Input: part model. Units: mm. Frame: model coordinates. Face numbers are marked on the shaded views. A direction names the side the tool comes from. Coordinates: 2 decimals unless noted, no trailing zeros. Loops run counter-clockwise (first coordinate to the right, second up) from the corner with the lowest first, then second, coordinate; pieces in that order, holes last. Notation, with made-up numbers: (-27.75, 1) -> (-19.75, 1) arc R33 ccw to (-19.75, 32) -> close; hole circle Ø8 at (6.25, -22). An arc over 180 degrees is marked (long way). Put each result on its own line as item: value. Start each with the question number.
1) Contact query for flat-ended pins moving along their axis: P1, Ø1.5, axis at x = -1, z = 9, coming from the +Y side; P2, Ø2, axis at x = -4.5, z = 47.5, coming from the +Y side; P3, Ø2, axis at y = -81, z = 3.5, coming from the -X side; P4, Ø5, axis at x = -35.5, y = -44, coming from the +Z side. Output: stop coordinate, or through.
2) Cut plane B-B (x = 37.5). Return the cut outline in (y, z), plus the area to 3 significant figures.
3) Cut plane A-A (y = -36.5). Return the cut outline in (x, z), plus the area to 3 significant figures.
4) Material intervals for L1, parallel to X at y = -19, z = 28; L2, parallel to Z at x = -13, y = -70.5, sorted ascending.
5) Cut plane C-C (z = 6). Return the cut outline in (x, y).
6) Cut plane D-D (y = -55.5). Return the cut outline in (x, z).
7) Set-up query: the marked faces 1, 2 and 3. Return all of +Z, -Z, +X, -X, +Y, -Y with unobstructed straight access to the full face (end or side cutting, diameter ignored); none if empty.
from build123d import *

# Parameters (mm, degrees)
F0_W      = 100
F0_H      = 100
F1_DEPTH  = 100
F2_R      = 35
F3_DEPTH  = 70
F4_R      = 35
F5_DEPTH  = 70
F6_R      = 35
F7_DEPTH  = 70
F8_R      = 35
F9_DEPTH  = 70
F11_R     = 35
F12_DEPTH = 70
F13_R     = 35
F14_DEPTH = 25
F10_R     = 35
F15_DEPTH = 70
F17_D     = 5


with BuildPart() as f1:
    # F0 (on Front) → F1 (new body)
    with BuildSketch(Plane.XZ):
        with Locations((50, 50)):
            Rectangle(F0_W, F0_H)
    extrude(amount=F1_DEPTH)

    # F2 (on Top) → F3 (join)
    with BuildSketch(Plane.XY):
        with Locations((48.346177, -50.003812)):
            Circle(F2_R)
    extrude(amount=-F3_DEPTH)

    # F4 (on Top) → F5 (join)
    with BuildSketch(Plane.XY):
        with Locations((49.174994, -45.859754)):
            Circle(F4_R)
    extrude(amount=-F5_DEPTH)

    # F6 (on Top) → F7 (join)
    with BuildSketch(Plane.XY):
        with Locations((48.553377, -49.589396)):
            Circle(F6_R)
    extrude(amount=-F7_DEPTH)

    # F8 (on Top) → F9 (join)
    with BuildSketch(Plane.XY):
        with Locations((50.625414, -48.760593)):
            Circle(F8_R)
    extrude(amount=-F9_DEPTH)

    # F11 (on Top) → F12 (join)
    with BuildSketch(Plane.XY):
        with Locations((50.038069, -49.650535)):
            Circle(F11_R)
    extrude(amount=-F12_DEPTH)

    # F13 (on face) → F14 (join)
    with BuildSketch(Plane.XY.offset(100)):
        with Locations((49.716454, -51.418651)):
            Circle(F13_R)
    extrude(amount=-F14_DEPTH)

    # F10 (on Right) → F15 (join)
    with BuildSketch(Plane.YZ):
        with Locations((-52.281633, 49.393684)):
            Circle(F10_R)
    extrude(amount=-F15_DEPTH)

    # F17 (through all)
    with Locations(Plane.XZ.offset(100)):
        with Locations((50.875958, 50.418209)):
            Hole(F17_D / 2)


solid = f1.part
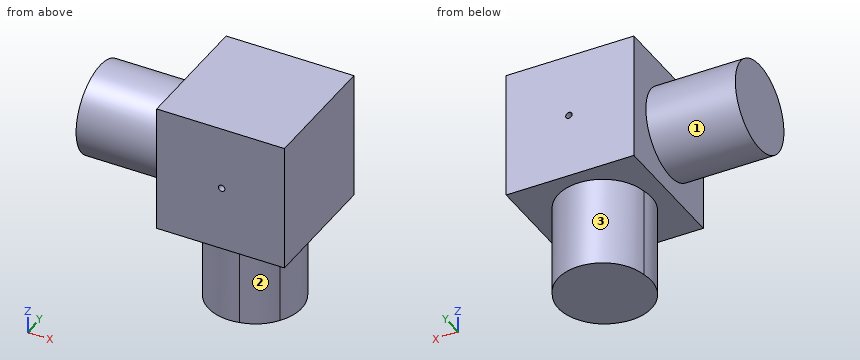
Results found:
1. P1: passes through
1. P2: stops at y = -17.29
1. P3: stops at x = 0
1. P4: stops at z = 83.91
2. outline: (-100, 0) -> (-83.28, 0) -> (-83.28, -70) -> (-12.86, -70) -> (-12.86, 0) -> (0, 0) -> (0, 100) -> (-100, 100) -> close
2. area: 14,900 mm2
3. outline: (-70, 18.15) -> (0, 18.15) -> (0, 0) -> (15.45, 0) -> (15.45, -70) -> (83.41, -70) -> (83.41, 0) -> (100, 0) -> (100, 100) -> (0, 100) -> (0, 80.63) -> (-70, 80.63) -> close; hole circle Ø5 at (50.88, 50.42)
3. area: 19,100 mm2
4. L1: x = 0 to 100
4. L2: z = 19.51 to 79.28
5. outline: (0, -100) -> (100, -100) -> (100, 0) -> (0, 0) -> close
6. outline: (-70, 14.54) -> (0, 14.54) -> (0, 0) -> (13.78, 0) -> (13.78, -70) -> (84.97, -70) -> (84.97, 0) -> (100, 0) -> (100, 100) -> (0, 100) -> (0, 84.25) -> (-70, 84.25) -> close; hole circle Ø5 at (50.88, 50.42)
7. face 1: -X
7. face 2: -Z, +X, -Y
7. face 3: -Z, +Y
